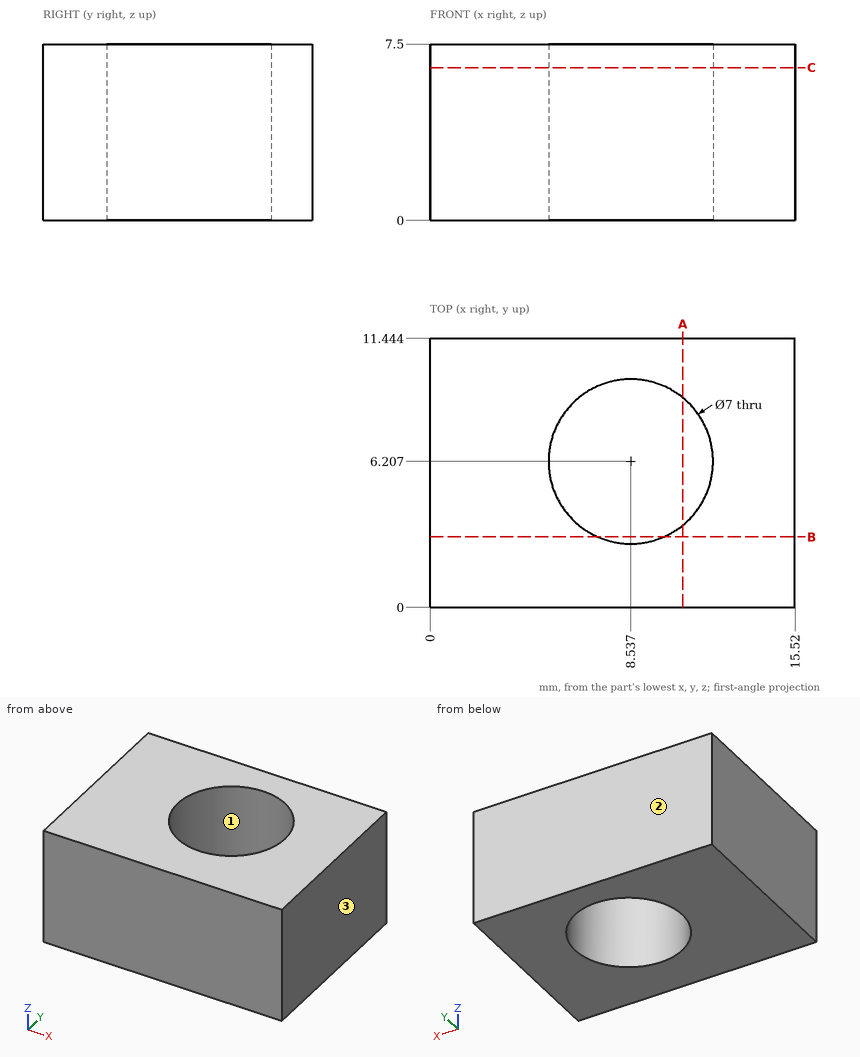
The drawing under review shows one solid part. Ordinate dimensions are in mm from its lowest x, y, z. Coordinates: 2 decimals unless noted, no trailing zeros. Write each loop counter-clockwise with the first axis right and the second up, starting at its lowest first coordinate (ties: lowest second). Pieces come first, ordered by that corner, then holes. Notation, with made-up numbers: (20.25, 32) - (56.25, 32) arc R28 ccw to (56.25, 68) - close; hole circle Ø3 at (25.25, 23). An arc over 180 degrees is marked (long way). Answer in a Markdown table with one row per item. Add a question column.
Q1. We need section A-A, the plane x = 10.75. State the section outline as (y, z) points (1 decimal).
Q2. We need section B-B, the plane y = 3. State the section outline as (x, z) points (1 decimal).
Q3. We need section C-C, the plane z = 6.5. State the section outline as (x, y) points, and give its area (3 significant figures).
Q4. For probe 1 along X at (y, z) = (6.25, 2.25); probe 2 along Y at (x, z) = (8, 4.5) (1 decimal); probe 3 along Y at (x, z) = (10.5, 0.75) (1 decimal), list the stretches that pass through material, from the lowest coordinate up.
Q5. Draft analysis for pull direction Y (two halves, no side actions). For the marked faces 1, 2 and 3, state which applies: +Y half, -Y half, draft (parallel to the pull), parting line (faces both ways), or undercut.
Q6. For P1, Ø1.5, axis at x = 7, y = 2, coming from the -Z side; P2, Ø4, axis at x = 8.54, y = 6.21, coming from the -Z side, all flat-tipped, find the tip position at first contact; note any pin that passes through.
Answer list:
| question | item | result |
|---|---|---|
| 1 | outline | (0, 0) - (3.5, 0) - (3.5, 7.5) - (0, 7.5) - close; (8.9, 0) - (11.4, 0) - (11.4, 7.5) - (8.9, 7.5) - close |
| 2 | outline | (0, 0) - (7.1, 0) - (7.1, 7.5) - (0, 7.5) - close; (9.9, 0) - (15.5, 0) - (15.5, 7.5) - (9.9, 7.5) - close |
| 3 | outline | (0, 0) - (15.52, 0) - (15.52, 11.44) - (0, 11.44) - close; hole circle Ø7 at (8.54, 6.21) |
| 3 | area | 139 mm2 |
| 4 | probe 1 | x = 0 to 5.04, 12.04 to 15.52 |
| 4 | probe 2 | y = 0 to 2.7, 9.7 to 11.4 |
| 4 | probe 3 | y = 0 to 3.3, 9.1 to 11.4 |
| 5 | face 1 | undercut |
| 5 | face 2 | +Y half |
| 5 | face 3 | draft |
| 6 | P1 | stops at z = 0 |
| 6 | P2 | passes through |
